Print and shaded views of the part. All mm, measured from the part's lowest x, y and z. Give positions to 0.01 mm unless a question says otherwise; leave off trailing zeros. Loops run counter-clockwise (first coordinate to the right, second up) from the corner with the lowest first, then second, coordinate; pieces in that order, holes last. Notation, with made-up numbers: M 7,-12.5 L 53,-12.5 A19 cw 53,3.5 Z; hole C -10,-35 d11. An arc over 180 degrees is marked long. Answer in a Markdown table with one row per item.
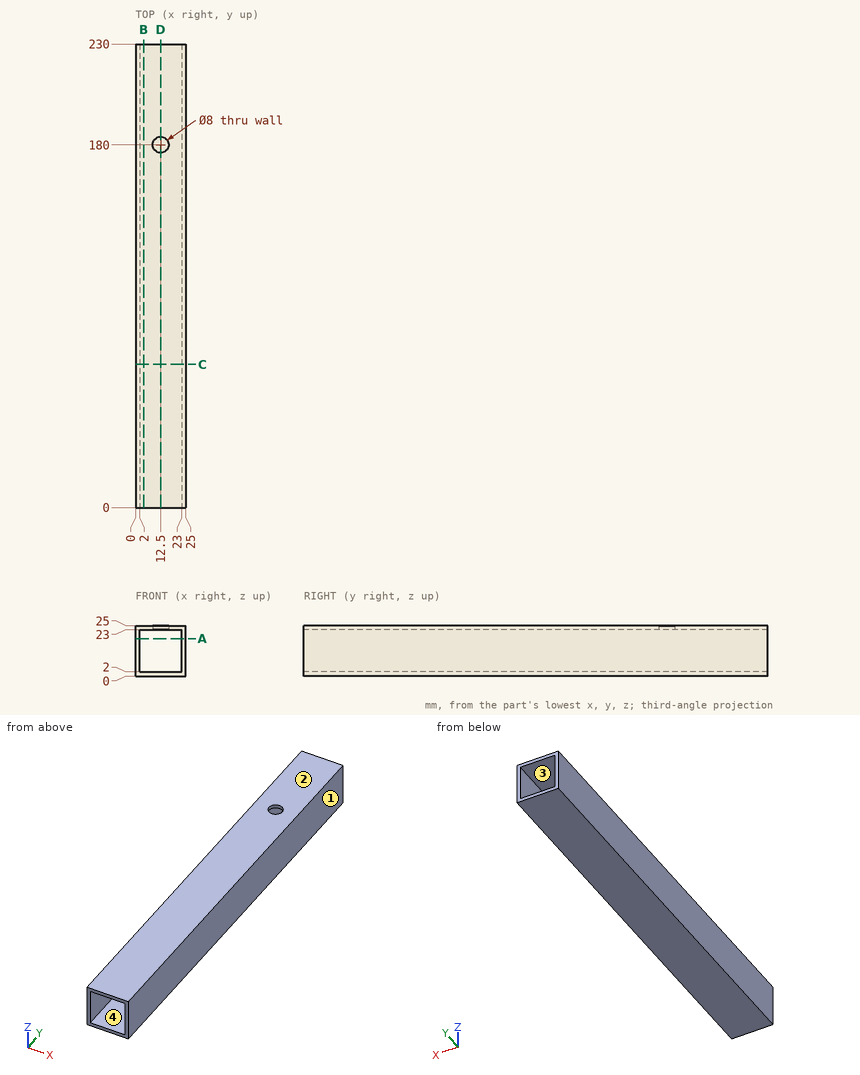
(1) Saw through at B-B, the plane x = 4. Give the cut face in (y, z).
Established:
| item | result |
|---|---|
| outline | M 0,0 L 230,0 L 230,2 L 0,2 Z; M 0,23 L 230,23 L 230,25 L 0,25 Z |
(2) Saw through at D-D, the plane x = 12.5. Give the cut face in (y, z).
Established:
| item | result |
|---|---|
| outline | M 0,0 L 230,0 L 230,2 L 0,2 Z; M 0,23 L 176,23 L 176,25 L 0,25 Z; M 184,23 L 230,23 L 230,25 L 184,25 Z |
(3) Saw through at C-C, the plane y = 71. Give the cut face in (x, z).
Established:
| item | result |
|---|---|
| outline | M 0,0 L 25,0 L 25,25 L 0,25 Z; hole M 2,2 L 23,2 L 23,23 L 2,23 Z |
(4) Saw through at A-A, the plane z = 18.5. Give the cut face in (x, y), and give its area (3 significant figures).
Established:
| item | result |
|---|---|
| outline | M 0,0 L 2,0 L 2,230 L 0,230 Z; M 23,0 L 25,0 L 25,230 L 23,230 Z |
| area | 920 mm2 |
(5) Mould opens along Z. For the marked faces 1, 2, 3 and 4 say: pulls with the +Z half, pulls with the -Z half, needs draft (parallel to the pull), parting line crosses it, or undercut.
Established:
| item | result |
|---|---|
| face 1 | needs draft |
| face 2 | pulls with the +Z half |
| face 3 | undercut |
| face 4 | undercut |
(6) Wall check: L1, parallel to Z at x = 19, y = 22; L2, parallel to Y at x = 12.5, z = 24.4. Give the ranges that are in metal, low to high.
Established:
| item | result |
|---|---|
| L1 | z = 0 to 2, 23 to 25 |
| L2 | y = 0 to 176, 184 to 230 |
